from build123d import *

# Parameters (mm, degrees)
BOSS_EXTRUDE1_DEPTH = 3.175
FILLET1_R           = 45.72
FILLET4_R           = 127
FILLET5_R           = 6.35
FILLET6_R           = 6.35
FILLET7_R           = 6.35
FILLET8_R           = 6.35
SKETCH4_R           = 14.2875
CUT_EXTRUDE1_DEPTH  = 18.415


with BuildPart() as part:
    # Sketch1 → Boss-Extrude1 (new body)
    with BuildSketch(Plane.XY):
        Polygon((0, 0), (165.1, 0), (165.1, 50.8), (-8.578307929, 50.8), (-173.494021533, -15.063128689), (-151.393719418, -65.863128689), align=None)
    extrude(amount=BOSS_EXTRUDE1_DEPTH)

    # Fillet1
    fillet1_edges = [part.edges().sort_by_distance(p)[0] for p in [
        (0, 0, 1.5875),
    ]]
    fillet(fillet1_edges, radius=FILLET1_R)

    # Fillet4
    fillet4_edges = [part.edges().sort_by_distance(p)[0] for p in [
        (-8.578307929, 50.8, 1.5875),
    ]]
    fillet(fillet4_edges, radius=FILLET4_R)

    # Fillet5
    fillet5_edges = [part.edges().sort_by_distance(p)[0] for p in [
        (-151.393719418, -65.863128689, 1.5875),
    ]]
    fillet(fillet5_edges, radius=FILLET5_R)

    # Fillet6
    fillet6_edges = [part.edges().sort_by_distance(p)[0] for p in [
        (-173.494021533, -15.063128689, 1.5875),
    ]]
    fillet(fillet6_edges, radius=FILLET6_R)

    # Fillet7
    fillet7_edges = [part.edges().sort_by_distance(p)[0] for p in [
        (165.1, 0, 1.5875),
    ]]
    fillet(fillet7_edges, radius=FILLET7_R)

    # Fillet8
    fillet8_edges = [part.edges().sort_by_distance(p)[0] for p in [
        (165.1, 50.8, 1.5875),
    ]]
    fillet(fillet8_edges, radius=FILLET8_R)

    # Sketch4 → Cut-Extrude1 (cut)
    with BuildSketch(Plane(origin=(0, 0, 0), x_dir=(-1, 0, 0), z_dir=(0, 0, -1))):
        with Locations((-141.674387764, 25.4)):
            Circle(SKETCH4_R)
        with Locations((134.369201797, -28.767007742)):
            Circle(SKETCH4_R)
        with Locations((3.969661405, 23.777990081)):
            Circle(SKETCH4_R)
    extrude(amount=-CUT_EXTRUDE1_DEPTH, mode=Mode.SUBTRACT)


solid = part.part
The model under review builds one solid part; all positions refer to its coordinate system, in mm. Round coordinates to 2 decimals unless told otherwise and drop trailing zeros. Order: outer loops, then holes, each group sorted by start corner. A loop starts at its lowest first (then second) coordinate and runs counter-clockwise, first axis right, second up. Notation, with made-up numbers: (81.25, 18) -> (114.25, 18) arc R18 cw to (114.25, 29) -> close; hole circle Ø1 at (-1.75, 61). An arc over 180 degrees is marked (long way). Use CSV: the item, a comma, the result in double quotes. Start each with the question number.
(1) Insertion check: pin 1 (1 mm diameter, centred on x = 42.5, z = 0.5, fed in from -Y). The pin has a flat end and moves straight along its axis. Give the tip position at first contact, or say it passes through.
(2) Mouldability with a two-part tool opening along X and no side actions: class faces 1 (the face through (-78.11, -33.98, 1.57)), 2 (the face through (-6, 7, 0)), 3 (the face through (-7.807, 48.578, 1.61)), 4 (the face through (128.476, 19.928, 1.565)) as pulls with the +X half, pulls with the -X half, needs draft (parallel to the pull), parting line crosses it, or undercut.
(3) Wall thickness on probe 1 along Y at (x, z) = (81.5, 2.4); probe 2 along X at (y, z) = (-25.5, 0.7); probe 3 along X at (y, z) = (-35, 1.5): over which ranges is each line inside the solid? List them lowest first. Write a range as from..to.
(4) Consider section A-A on z = 1.15. State how many separate pieces and enclosed holes the cut face has, and give its area (3 significant figures).
(5) Consider section C-C on x = -85. Write out the cut boundary in (y, z) (3 decimals).
(6) Consider section B-B on x = 85. Write out the cut boundary in (y, z) (3 decimals).
Responses:
1,pin 1,"y = 0"
2,face 1,"pulls with the +X half"
2,face 2,"needs draft"
2,face 3,"pulls with the -X half"
2,face 4,"undercut"
3,probe 1,"0..50.8"
3,probe 2,"-168.95..-148.28, -120.46..-58.61"
3,probe 3,"-164.82..-147.23, -121.51..-80.45"
4,separate pieces,"1"
4,enclosed holes,"3"
4,area,"15,700 mm²"
5,outline,"(-36.979, 0) -> (20.279, 0) -> (20.279, 3.175) -> (-36.979, 3.175) -> close"
6,outline,"(0, 0) -> (50.8, 0) -> (50.8, 3.175) -> (0, 3.175) -> close"
